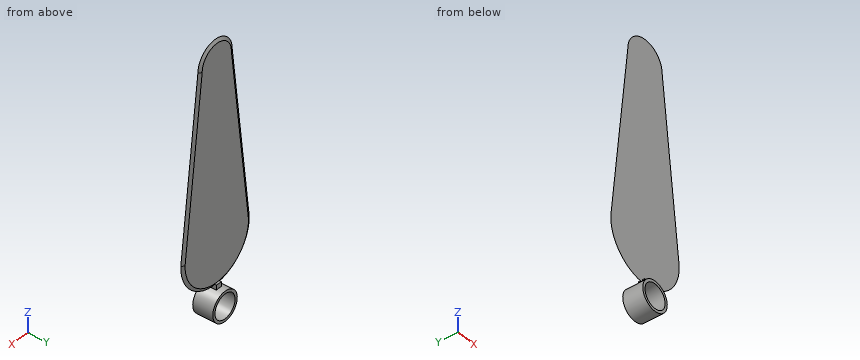
from build123d import *

# Parameters (mm, degrees)
SALIENTE_EXTRUIR1_DEPTH      = 0.3
SALIENTE_EXTRUIR1_TAPER      = 60
CROQUIS3_W                   = 1
CROQUIS3_H                   = 1
SALIENTE_EXTRUIR2_DEPTH      = 0.3
CROQUIS4_W                   = 1
CROQUIS4_H                   = 1
SALIENTE_EXTRUIR3_DEPTH      = 0.519615
SALIENTE_EXTRUIR4_DEPTH      = 1.7
SALIENTE_EXTRUIR4_DEPTH_BACK = 1.7
CROQUIS5_R                   = 2.5
CROQUIS7_R                   = 2.05
CORTAR_EXTRUIR1_DEPTH        = 43.960206994


with BuildPart() as part:
    # Croquis1 → Saliente-Extruir1 (new body)
    with BuildSketch(Plane(origin=(0, 0, 0), x_dir=(1, 0, 0), z_dir=(0, 1, 0))):
        with BuildLine():
            ThreePointArc((-3.5, 0), (0, -3.5), (3.5, 0))
            Line((3.5, 0), (6.998354756, 29.848241299))
            ThreePointArc((6.998354756, 29.848241299), (0, 37), (-6.998354756, 29.848241299))
            Line((-6.998354756, 29.848241299), (-3.5, 0))
        make_face()
    extrude(amount=SALIENTE_EXTRUIR1_DEPTH, taper=SALIENTE_EXTRUIR1_TAPER)



with BuildPart() as body_2:
    # Croquis3 → Saliente-Extruir2 (new body)
    with BuildSketch(Plane.XY.offset(-37)):
        with Locations((0, 0.15)):
            Rectangle(CROQUIS3_W, CROQUIS3_H)
    extrude(amount=-SALIENTE_EXTRUIR2_DEPTH)


with BuildPart() as part_1:
    add(part.part)

    add(body_2.part)  # Saliente-Extruir3 merges body 2
    # Croquis4 → Saliente-Extruir3 (add)
    with BuildSketch(Plane.XY.offset(-37)):
        with Locations((0, 0.15)):
            Rectangle(CROQUIS4_W, CROQUIS4_H)
    extrude(amount=SALIENTE_EXTRUIR3_DEPTH)

    # Croquis5 → Saliente-Extruir4 (add, two sides: drawn at the far end of the back side and taken through both)
    with BuildSketch(Plane(origin=(0, 0, 0), x_dir=(1, 0, 0), z_dir=(0, 1, 0)).offset(-SALIENTE_EXTRUIR4_DEPTH_BACK)):
        with Locations(Location((0, 39.749489743, 0), (0, 0, 270))):
            Circle(CROQUIS5_R)
    extrude(amount=SALIENTE_EXTRUIR4_DEPTH + SALIENTE_EXTRUIR4_DEPTH_BACK)

    # Croquis7 → Cortar-Extruir1 (cut, through all)
    with BuildSketch(Plane(origin=(0, 1.7, 0), x_dir=(1, 0, 0), z_dir=(0, 1, 0))):
        with Locations(Location((0, 39.749489743, 0), (0, 0, 270))):
            Circle(CROQUIS7_R)
    extrude(amount=-CORTAR_EXTRUIR1_DEPTH, mode=Mode.SUBTRACT)


solid = part_1.part
Could you check a few things on this model? Use its own coordinates, in mm. Give positions to 0.01 mm unless a question says otherwise; leave off trailing zeros. Order: outer loops, then holes, each group sorted by start corner. A loop starts at its lowest first (then second) coordinate and runs counter-clockwise, first axis right, second up. Notation, with made-up numbers: (61.25, 34) - (108.25, 34) arc R18 ccw to (108.25, 46) - close; hole circle Ø6 at (57, -22.75). An arc over 180 degrees is marked (long way). Return JSON: item names as keys, results as strings. Group by question number.
Q1. Will these pins go through, and if not, where does the flat tip stop? pin 1 Ø1.5 at (y, z) = (1, -8) entering from +X; pin 2 Ø0.7 at (y, z) = (0, -36.5) entering from -X; pin 3 Ø7 at (x, z) = (1, -16.5) entering from -Y.
Q2. Suppose I cut it at A-A, the plane y = 1.1. Please give me the cut outline in (x, z).
Q3. Please list where these lines run through material, in increasing order: line 1 along Y through (x, z) = (3.5, -9); line 2 along X through (y, z) = (0.25, -6); line 3 along Z through (x, y) = (-1, -1.4). Write a range as [from, to].
Resolved:
{
 "1": {"pin 1": "stops at x = 4", "pin 2": "stops at x = -3.34", "pin 3": "stops at y = 0"},
 "2": {"outline": "circle Ø5 at (0, -39.75); hole circle Ø4.1 at (0, -39.75)"},
 "3": {"line 1": "y = [0, 0.3]", "line 2": "x = [-3.77, 3.77]", "line 3": "z = [-42.04, -41.54], [-37.96, -37.46]"}
}
